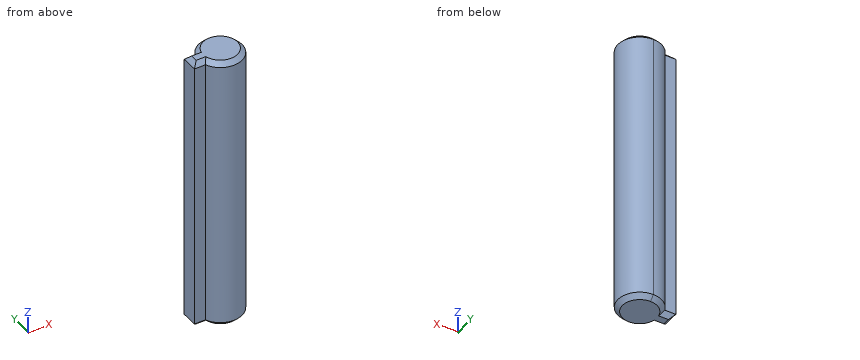
from build123d import *

# Parameters (mm, degrees)
BOSS_EXTRUDE1_DEPTH = 62
CHAMFER1_SIZE       = 1
CHAMFER2_SIZE       = 1
SCALE1_SCALE        = 0.75
SCALE2_SCALE        = 0.85


with BuildPart() as part:
    # Sketch1 → Boss-Extrude1 (new body)
    with BuildSketch(Plane(origin=(0, 0, 0), x_dir=(0, 1, 0), z_dir=(0, 0, 1))):
        with BuildLine():
            Line((1.8, 6.897570975), (-1.8, 6.897570975))
            Line((-1.8, 6.897570975), (-1.8, 4.449719092))
            ThreePointArc((-1.8, 4.449719092), (0, 4.8), (1.8, 4.449719092))
            Line((1.8, 4.449719092), (1.8, 6.897570975))
        make_face()
        with BuildLine():
            ThreePointArc((1.8, 4.449719092), (0, 4.8), (-1.8, 4.449719092))
            Line((-1.8, 4.449719092), (-1.8, 1.697570975))
            Line((-1.8, 1.697570975), (1.8, 1.697570975))
            Line((1.8, 1.697570975), (1.8, 4.449719092))
        make_face()
        with BuildLine():
            Line((-1.8, 1.697570975), (-1.8, 4.449719092))
            ThreePointArc((-1.8, 4.449719092), (-2.683281573, -3.979949748), (4.8, 0))
            ThreePointArc((4.8, 0), (3.979949748, 2.683281573), (1.8, 4.449719092))
            Line((1.8, 4.449719092), (1.8, 1.697570975))
            Line((1.8, 1.697570975), (-1.8, 1.697570975))
        make_face()
    extrude(amount=BOSS_EXTRUDE1_DEPTH)

    # Chamfer1
    chamfer1_edges = [part.edges().sort_by_distance(p)[0] for p in [
        (3.979949748, -2.683281573, 62),
        (-5.673645034, 1.8, 62),
        (-6.897570975, 0, 62),
        (-5.673645034, -1.8, 62),
    ]]
    chamfer(chamfer1_edges, length=CHAMFER1_SIZE)

    # Chamfer2
    chamfer2_edges = [part.edges().sort_by_distance(p)[0] for p in [
        (-6.897570975, 0, 0),
        (-5.673645034, 1.8, 0),
        (3.979949748, -2.683281573, 0),
        (-5.673645034, -1.8, 0),
    ]]
    chamfer(chamfer2_edges, length=CHAMFER2_SIZE)


with BuildPart() as part_1:
    # Scale1: scaled about (-0.57130559, 0, 31)
    add(part.part.scale(SCALE1_SCALE).moved(Location((-0.142826398, 0, 7.75))))


with BuildPart() as part_2:
    # Scale2: scaled about (-0.57130559, 0, 31)
    add(part_1.part.scale(SCALE2_SCALE).moved(Location((-0.085695839, 0, 4.65))))


solid = part_2.part
Check sheet for the modelled part. Datum: model origin and axes. Units: mm. Give positions to 0.01 mm unless a question says otherwise; leave off trailing zeros. Write each loop counter-clockwise with the first axis right and the second up, starting at its lowest first coordinate (ties: lowest second). Pieces come first, ordered by that corner, then holes. Notation, with made-up numbers: M 64.25,-29.75 L 108.25,-29.75 A23 cw 108.25,-20.75 Z; hole C -1,-36.75 d10. An arc over 180 degrees is marked long. Use one line per item in the form item = value.
(1) Depth check by flat-ended pin: P1, Ø0.5, axis at x = -3.5, z = 29, coming from the -Y side; P2, Ø2, axis at x = -3, z = 25, coming from the -Y side; P3, Ø1, axis at x = -1.5, z = 36.5, coming from the +Y side. Enter the tip coordinate at first touch or a pass-through.
Answer block:
P1 = -1.15
P2 = -2.48
P3 = 2.96
(2) Section check A-A on z = 16. Record the boundary of the cut face in (x, y).
Answer block:
outline = M -4.6,-1.15 L -3.04,-1.15 A3.06 ccw long -3.04,1.15 L -4.6,1.15 Z
(3) Material ranges on line 1 along Y through (x, z) = (-3.75, 43); line 2 along Y through (x, z) = (-3, 38); line 3 along X through (y, z) = (1.5, 36.5), recorded low to high.
Answer block:
line_1 = -1.15 to 1.15
line_2 = -1.25 to 1.25
line_3 = -2.87 to 2.46
